Model file for the job. Use its own axes, mm. A direction names the side the tool comes from. Give positions to 0.01 mm unless a question says otherwise; leave off trailing zeros. Loops run counter-clockwise (first coordinate to the right, second up) from the corner with the lowest first, then second, coordinate; pieces in that order, holes last. Notation, with made-up numbers: (36, 60.5) - (82, 60.5) arc R33 cw to (82, 92.5) - close; hole circle Ø1 at (13.5, 75). An arc over 180 degrees is marked (long way). Use a Markdown table: item, result.
from build123d import *

# Parameters (mm, degrees)
F0_R     = 4
F0_R_2   = 7.5
F1_DEPTH = 4
F2_DEPTH = 60


with BuildPart() as f1:
    # F0 (on Front) → F1 (new body)
    with BuildSketch(Plane.XZ):
        with BuildLine():
            ThreePointArc((2.14326, -24.907959), (18.419847, -16.902936), (25, 0))
            ThreePointArc((25, 0), (18.059137, 17.287787), (1.090594, 24.976201))
            ThreePointArc((1.090594, 24.976201), (-24.994436, -0.527438), (2.14326, -24.907959))
        make_face()
        Circle(F0_R, mode=Mode.SUBTRACT)
        with BuildLine():
            ThreePointArc((1.090594, 24.976201), (18.059137, 17.287787), (25, 0))
            ThreePointArc((25, 0), (18.419847, -16.902936), (2.14326, -24.907959))
            Line((2.14326, -24.907959), (171.200226, -10.361081))
            ThreePointArc((171.200226, -10.361081), (156.003116, 3.292011), (170.610733, 17.574048))
            Line((170.610733, 17.574048), (1.090594, 24.976201))
        make_face()
        with BuildLine():
            ThreePointArc((184, 3.587376), (180.113117, 13.268537), (170.610733, 17.574048))
            ThreePointArc((170.610733, 17.574048), (156.003116, 3.292011), (171.200226, -10.361081))
            ThreePointArc((171.200226, -10.361081), (180.315114, -5.878268), (184, 3.587376))
        make_face()
        with Locations((170, 3.587376)):
            Circle(F0_R_2, mode=Mode.SUBTRACT)
        with Locations((170, 3.587376)):
            Circle(F0_R_2)
    extrude(amount=-F1_DEPTH)

    # F0 (on Front) → F2 (join)
    with BuildSketch(Plane.XZ):
        with Locations((170, 3.587376)):
            Circle(F0_R_2)
    extrude(amount=F2_DEPTH)


solid = f1.part
(1) Slice it at C-C, the plane x = 25. Write the cut outline in (y, z).
Computed:
| item | result |
|---|---|
| outline | (0, -22.94) - (4, -22.94) - (4, 23.93) - (0, 23.93) - close |
(2) Slice it at D-D, the plane z = -16. Write the cut outline in (x, y).
Computed:
| item | result |
|---|---|
| outline | (-19.21, 0) - (105.67, 0) - (105.67, 4) - (-19.21, 4) - close |
(3) Pin check, flat tips, straight feed: P1, Ø6, axis at x = 147.5, z = -16, coming from the +Y side; P2, Ø8, axis at y = -41.5, z = 8.5, coming from the +X side; P3, Ø10, axis at x = 14.5, z = -7.5, coming from the -Y side; P4, Ø4, axis at y = -42.5, z = 7.5, coming from the -X side. Stop position of each tip, or through.
Computed:
| item | result |
|---|---|
| P1 | through |
| P2 | x = 177.44 |
| P3 | y = 0 |
| P4 | x = 162.75 |
(4) Slice it at A-A, the plane z = 0. Write the cut outline in (x, y).
Computed:
| item | result |
|---|---|
| outline | (-25, 0) - (-4, 0) - (-4, 4) - (-25, 4) - close; (4, 0) - (163.41, 0) - (163.41, -60) - (176.59, -60) - (176.59, 0) - (183.53, 0) - (183.53, 4) - (4, 4) - close |
(5) Drill centre lines: probe 1 along Z at (x, y) = (0, 3.05); probe 2 along Y at (x, z) = (58, -8.5); probe 3 along X at (y, z) = (-41, 2.5). Where is each one in solid material? Low to high. Write a range as [from, to].
Computed:
| item | result |
|---|---|
| probe 1 | [-25, -4], [4, 25] |
| probe 2 | [0, 4] |
| probe 3 | [162.58, 177.42] |
(6) Slice it at B-B, the plane y = -38. Write the cut outline in (x, z), plus the area to 3 significant figures.
Computed:
| item | result |
|---|---|
| outline | circle Ø15 at (170, 3.59) |
| area | 177 mm² |
(7) 3-axis set-ups, long thin cutter, end or side, ignore diameter. For faces 1 (the cylindrical face through (177.154, -29.58, 5.84)), 2 (the flat face through (85.488, 1.972, -17.736)): which of +Z, -Z, +X, -X, +Y, -Y reach the whole face in a straight line?
Computed:
| item | result |
|---|---|
| face 1 | -Y |
| face 2 | -Z, +X, +Y, -Y |
